Here's how the part is built. I have some questions about the finished solid (model axes, mm). A direction names the side the tool comes from. Give positions to 0.01 mm unless a question says otherwise; leave off trailing zeros. Order: outer loops, then holes, each group sorted by start corner. A loop starts at its lowest first (then second) coordinate and runs counter-clockwise, first axis right, second up. Notation, with made-up numbers: (80.25, 23) -> (100.25, 23) arc R20 ccw to (100.25, 52) -> close; hole circle Ø6 at (42, 13). An arc over 180 degrees is marked (long way). Write each question's results on one line, items separated by ' | '. Start each with the question number.
Q1. I need wall thicknesses on line 1 along Z through (x, y) = (14, -95); line 2 along Y through (x, z) = (13.5, 42.5); line 3 along Y through (x, z) = (8.5, 39). Which ranges of each line are inside material? Lowest first, please. Write a range as [from, to].
Q2. For faces 1 (the face through (8, -91, 7.087)), 2 (the face through (16, 110.259, 25)), which set-ups out of +Z, -Z, +X, -X, +Y, -Y let a thin tool reach every point of the face, with its end or its side?
Q3. Imagine slicing it at A-A, the plane z = 20. Please give me the cut outline in (x, y).
Q4. I'm going to push flat-ended pins straight in: pin 1 (5 mm diameter, centred on y = -84, z = 9.5, fed in from +X); pin 2 (1.5 mm diameter, centred on x = 21, z = 39.5, fed in from -Y); pin 3 (10 mm diameter, centred on x = 11, y = -95.5, fed in from +Z). Where does each tip first touch, or does it pass through?
Q5. Imagine slicing it at C-C, the plane z = 33.5. Please give me the cut outline in (x, y), then the cut area to 3 significant figures.
Q6. Imagine slicing it at B-B, the plane y = -39. Please give me the cut outline in (x, z), then the cut area to 3 significant figures.
Q7. Imagine slicing it at D-D, the plane y = -9.5. Please give me the cut outline in (x, z), then the cut area to 3 significant figures.
```python
from build123d import *

# Parameters (mm, degrees)
F1_DEPTH = 50
F3_DEPTH = 32.5
F4_R     = 50


with BuildPart() as f1:
    # F0 (on Top) → F1 (new body)
    with BuildSketch(Plane.XY):
        with BuildLine():
            Line((32.5, 110.258812), (0, 110.258812))
            Line((0, 110.258812), (0, -112.741188))
            Line((0, -112.741188), (9, -112.741188))
            ThreePointArc((9, -112.741188), (26.579848, -47.271274), (32.5, 20.258812))
            Line((32.5, 20.258812), (32.5, 110.258812))
        make_face()
    extrude(amount=F1_DEPTH)

    # F2 (on face) → F3 (cut)
    with BuildSketch(Plane(origin=(0, 0, 0), x_dir=(0, -1, 0), z_dir=(-1, 0, 0))):
        with BuildLine():
            Line((-37.258812, 50), (-36.241843, 50))
            ThreePointArc((-36.241843, 50), (-36.750328, 50.001724), (-37.258812, 50))
        make_face()
        with BuildLine():
            Line((112.741188, 50), (-12.258812, 50))
            Line((-12.258812, 50), (-36.241843, 50))
            ThreePointArc((-36.241843, 50), (-20.898034, 48.307281), (-6.225791, 43.509042))
            ThreePointArc((-6.225791, 43.509042), (31.978225, 16.584949), (77.741188, 7.087324))
            Line((77.741188, 7.087324), (112.741188, 7.087324))
            Line((112.741188, 7.087324), (112.741188, 50))
        make_face()
    extrude(amount=-F3_DEPTH, mode=Mode.SUBTRACT)

    # F4
    f4_edges = [f1.edges().sort_by_distance(p)[0] for p in [
        (16.12311, 6.225791, 43.509042),
    ]]
    fillet(f4_edges, radius=F4_R)


solid = f1.part
```
Geometry check:
1) line 1: [0, 7.09] | line 2: [7.07, 110.26] | line 3: [2.01, 110.26]
2) face 1: +Z, +X, -X, -Y | face 2: +Z, -Z, +X, -X, +Y
3) outline: (0, -24.8) -> (29.88, -24.8) arc R388.11 ccw to (32.5, 20.26) -> (32.5, 110.26) -> (0, 110.26) -> close
4) pin 1: x = 18.42 | pin 2: y = 1.69 | pin 3: z = 7.09
5) outline: (0, -4.41) -> (31.72, -4.41) arc R388.11 ccw to (32.5, 20.26) -> (32.5, 110.26) -> (0, 110.26) -> close | area: 3,720 mm²
6) outline: (0, 0) -> (27.95, 0) -> (27.95, 13.81) -> (0, 13.81) -> close | area: 386 mm²
7) outline: (0, 0) -> (31.36, 0) -> (31.36, 29.52) -> (0, 29.52) -> close | area: 926 mm²
